```python
from build123d import *

# Parameters (mm, degrees)
F1_DEPTH     = 2.54
F2_T1_DEPTH  = 116.3302767053
F2_T3_DEPTH  = 79.5286740138
F2_T5_DEPTH  = 45.6964583098
F2_T10_DEPTH = 61.1019260212
F2_T15_DEPTH = 53.0222754018
F2_T20_DEPTH = 50.3447363809
F2_T25_DEPTH = 59.0101457163
F2_T31_DEPTH = 50.1034033931
F2_T35_DEPTH = 53.0222754018
F2_T42_DEPTH = 50.3447363809
F2_T46_DEPTH = 48.0116230882


# Not quite as in the source:
# - a fillet or chamfer that OpenCascade refuses, or shapes differently, is made with other operations: its cross-section is extruded or revolved along the edge and cut away or added


with BuildPart() as f1:
    # F0 (on Front) → F1 (new body)
    with BuildSketch(Plane.XZ):
        Polygon((67.8614974022, 19.1138908267), (-26.4717340469, 19.1138908267), (-26.4717340469, -38.417737931), (12.6331467181, -38.417737931), (30.848396942, -38.417737931), (67.8614974022, -38.417737931), align=None)
        Polygon((30.848396942, -38.417737931), (12.6331467181, -38.417737931), (-4.6027889475, -64.2147809267), (19.0966241062, -64.2147809267), align=None)
    extrude(amount=F1_DEPTH)

    # F2: fillet of radius 5.08 on 8 edges, made by hand

    # F2_s2 → F2_t1 (cut)
    with BuildSketch(Plane.YZ.offset(-37.470256675)):
        with BuildLine():
            ThreePointArc((-2.54, 19.1138908267), (-0.6805909488, 17.2544817755), (0, 14.7144817755))
            Line((0, 14.7144817755), (0, 19.1138908267))
            Line((0, 19.1138908267), (-2.54, 19.1138908267))
        make_face()
    extrude(amount=F2_T1_DEPTH, mode=Mode.SUBTRACT)

    # F2_s4 → F2_t3 (cut)
    with BuildSketch(Plane.XY.offset(-49.4162605591)):
        with BuildLine():
            ThreePointArc((-26.4717340469, -2.54), (-24.6123249957, -0.6805909488), (-22.0723249957, 0))
            Line((-22.0723249957, 0), (-26.4717340469, 0))
            Line((-26.4717340469, 0), (-26.4717340469, -2.54))
        make_face()
        with BuildLine():
            ThreePointArc((67.8614974022, -2.54), (66.002088351, -0.6805909488), (63.462088351, 0))
            Line((63.462088351, 0), (67.8614974022, 0))
            Line((67.8614974022, 0), (67.8614974022, -2.54))
        make_face()
    extrude(amount=F2_T3_DEPTH, mode=Mode.SUBTRACT)

    # F2_s6 → F2_t5 (cut)
    with BuildSketch(Plane.YZ.offset(-15.6013115756)):
        with BuildLine():
            ThreePointArc((-2.54, -64.2147809267), (-0.6805909488, -62.3553718755), (0, -59.8153718755))
            Line((0, -59.8153718755), (0, -64.2147809267))
            Line((0, -64.2147809267), (-2.54, -64.2147809267))
        make_face()
    extrude(amount=F2_T5_DEPTH, mode=Mode.SUBTRACT)


with BuildPart() as f2_tool8:
    # F2_s9 → F2_t10 (new body)
    with BuildSketch(Plane.YZ.offset(-37.470256675)):
        with BuildLine():
            ThreePointArc((-2.54, -38.417737931), (-0.6805909488, -36.5583288798), (0, -34.0183288798))
            Line((0, -34.0183288798), (0, -38.417737931))
            Line((0, -38.417737931), (-2.54, -38.417737931))
        make_face()
    extrude(amount=F2_T10_DEPTH)

    split(bisect_by=Plane(origin=(26.480413057, 0, -17.6925198724), x_dir=(0, 1, 0), z_dir=(-0.8314859511, 0, 0.5555457795)), keep=Keep.TOP)


with BuildPart() as f1_1:
    add(f1.part)

    # F2_t7: cut F2_tool8
    add(f2_tool8.part, mode=Mode.SUBTRACT)


with BuildPart() as f2_tool13:
    # F2_s14 → F2_t15 (new body)
    with BuildSketch(Plane(origin=(-7.737083512, 0, -11.5801010106), x_dir=(0, 1, 0), z_dir=(-0.5555457795, 0, -0.8314859511))):
        with BuildLine():
            ThreePointArc((-2.54, 31.8470961801), (-0.6805909488, 33.7065052313), (0, 36.2465052313))
            Line((0, 36.2465052313), (0, 31.8470961801))
            Line((0, 31.8470961801), (-2.54, 31.8470961801))
        make_face()
    extrude(amount=F2_T15_DEPTH)

    split(bisect_by=Plane.XY.offset(-38.417737931), keep=Keep.BOTTOM)


with BuildPart() as f1_2:
    add(f1_1.part)

    # F2_t12: cut F2_tool13
    add(f2_tool13.part, mode=Mode.SUBTRACT)


with BuildPart() as f2_tool18:
    # F2_s19 → F2_t20 (new body)
    with BuildSketch(Plane(origin=(-25.5031201264, 0, -55.983475482), x_dir=(0, 1, 0), z_dir=(0.4145583774, 0, 0.9100227204))):
        with BuildLine():
            ThreePointArc((-2.54, -43.9991372067), (-0.6805909488, -42.1397281555), (0, -39.5997281555))
            Line((0, -39.5997281555), (0, -43.9991372067))
            Line((0, -43.9991372067), (-2.54, -43.9991372067))
        make_face()
    extrude(amount=F2_T20_DEPTH)

    split(bisect_by=Plane.XY.offset(-38.417737931), keep=Keep.BOTTOM)


with BuildPart() as f1_3:
    add(f1_2.part)

    # F2_t17: cut F2_tool18
    add(f2_tool18.part, mode=Mode.SUBTRACT)


with BuildPart() as f2_tool23:
    # F2_s24 → F2_t25 (new body)
    with BuildSketch(Plane.YZ.offset(19.849874314)):
        with BuildLine():
            ThreePointArc((-2.54, -38.417737931), (-0.6805909488, -36.5583288798), (0, -34.0183288798))
            Line((0, -34.0183288798), (0, -38.417737931))
            Line((0, -38.417737931), (-2.54, -38.417737931))
        make_face()
    extrude(amount=F2_T25_DEPTH)

    split(bisect_by=Plane(origin=(40.040214538, 0, -18.2402109276), x_dir=(0, 1, 0), z_dir=(0.9100227204, 0, -0.4145583774)), keep=Keep.TOP)


with BuildPart() as f1_4:
    add(f1_3.part)

    # F2_t22: cut F2_tool23
    add(f2_tool23.part, mode=Mode.SUBTRACT)


with BuildPart() as f2_tool29:
    # F2_s30 → F2_t31 (new body)
    with BuildSketch(Plane.YZ.offset(-26.4717340469)):
        with BuildLine():
            ThreePointArc((-2.54, -38.417737931), (-0.6805909488, -36.5583288798), (0, -34.0183288798))
            Line((0, -34.0183288798), (0, -38.417737931))
            Line((0, -38.417737931), (-2.54, -38.417737931))
        make_face()
    extrude(amount=F2_T31_DEPTH)

    split(bisect_by=Plane(origin=(26.480413057, 0, -17.6925198724), x_dir=(0, 1, 0), z_dir=(0.8314859511, 0, -0.5555457795)), keep=Keep.TOP)


with BuildPart() as f2_tool33:
    # F2_s34 → F2_t35 (new body)
    with BuildSketch(Plane(origin=(-7.737083512, 0, -11.5801010106), x_dir=(0, 1, 0), z_dir=(-0.5555457795, 0, -0.8314859511))):
        with BuildLine():
            ThreePointArc((-2.54, 31.8470961801), (-0.6805909488, 33.7065052313), (0, 36.2465052313))
            Line((0, 36.2465052313), (0, 31.8470961801))
            Line((0, 31.8470961801), (-2.54, 31.8470961801))
        make_face()
    extrude(amount=F2_T35_DEPTH)

    split(bisect_by=Plane.XY.offset(-38.417737931), keep=Keep.TOP)


with BuildPart() as f2_tool29_1:
    add(f2_tool29.part)

    # F2_t37: intersect F2_tool33
    add(f2_tool33.part, mode=Mode.INTERSECT)


with BuildPart() as f1_5:
    add(f1_4.part)

    # F2_t27: cut F2_tool29
    add(f2_tool29_1.part, mode=Mode.SUBTRACT)


with BuildPart() as f2_tool40:
    # F2_s41 → F2_t42 (new body)
    with BuildSketch(Plane(origin=(-25.5031201264, 0, -55.983475482), x_dir=(0, 1, 0), z_dir=(0.4145583774, 0, 0.9100227204))):
        with BuildLine():
            ThreePointArc((-2.54, -43.9991372067), (-0.6805909488, -42.1397281555), (0, -39.5997281555))
            Line((0, -39.5997281555), (0, -43.9991372067))
            Line((0, -43.9991372067), (-2.54, -43.9991372067))
        make_face()
    extrude(amount=F2_T42_DEPTH)

    split(bisect_by=Plane.XY.offset(-38.417737931), keep=Keep.TOP)


with BuildPart() as f2_tool44:
    # F2_s45 → F2_t46 (new body)
    with BuildSketch(Plane.YZ.offset(19.849874314)):
        with BuildLine():
            ThreePointArc((-2.54, -38.417737931), (-0.6805909488, -36.5583288798), (0, -34.0183288798))
            Line((0, -34.0183288798), (0, -38.417737931))
            Line((0, -38.417737931), (-2.54, -38.417737931))
        make_face()
    extrude(amount=F2_T46_DEPTH)

    split(bisect_by=Plane(origin=(40.040214538, 0, -18.2402109276), x_dir=(0, 1, 0), z_dir=(-0.9100227204, 0, 0.4145583774)), keep=Keep.TOP)


with BuildPart() as f2_tool40_1:
    add(f2_tool40.part)

    # F2_t48: intersect F2_tool44
    add(f2_tool44.part, mode=Mode.INTERSECT)


with BuildPart() as f1_6:
    add(f1_5.part)

    # F2_t38: cut F2_tool40
    add(f2_tool40_1.part, mode=Mode.SUBTRACT)


solid = f1_6.part
```
Can you work these out from the model? Positions are in its coordinate system, mm. A direction names the side the tool comes from. Coordinates: 2 decimals unless noted, no trailing zeros. Order: outer loops, then holes, each group sorted by start corner. A loop starts at its lowest first (then second) coordinate and runs counter-clockwise, first axis right, second up. Notation, with made-up numbers: (-7.75, 14) - (11.25, 14) arc R8 ccw to (11.25, 19) - close; hole circle Ø7 at (89, 11.25). An arc over 180 degrees is marked (long way). Answer in a Markdown table with one row per item.
1. Suppose I cut it at B-B (z = -28.5). Please give me the cut outline in (x, y), and give its area (3 significant figures).
Reply:
| item | result |
|---|---|
| outline | (-26.47, -2.54) - (67.86, -2.54) arc R5.08 ccw to (63.46, 0) - (-22.07, 0) arc R5.08 ccw to start |
| area | 233 mm^2 |
2. If I drill on line 1 along Z through (x, y) = (1.5, -2.25); line 2 along Z through (x, y) = (-4, -2.15); line 3 along X through (y, z) = (-0.6, -5.5), over which ranges is the centre line in solid material (lowest first)?
Reply:
| item | result |
|---|---|
| line 1 | z = -64.03 to -55.41, -38.24 to 18.93 |
| line 2 | z = -63.97 to -63.76, -38.17 to 18.86 |
| line 3 | x = -24.47 to 65.86 |
3. If we mould it in two halves opening along Z, with no side actions, what happens to faces 1 (the flat face through (20, 0, -14)), 2 (the cylindrical face through (47.66, -0.7, -36.59)), 3 (the cylindrical face through (7.97, -0.7, -48.68))? For each: pulls with the +Z half, pulls with the -Z half, needs draft (parallel to the pull), parting line crosses it, or undercut.
Reply:
| item | result |
|---|---|
| face 1 | needs draft |
| face 2 | pulls with the -Z half |
| face 3 | undercut |
4. Suppose I cut it at A-A (y = -0.7). Please give me the cut outline in (x, z).
Reply:
| item | result |
|---|---|
| outline | (-24.65, -36.59) - (16.05, -36.59) - (-1.19, -62.39) - (17.92, -62.39) - (29.67, -36.59) - (66.04, -36.59) - (66.04, 17.29) - (-24.65, 17.29) - close |
5. For faces 4 (the cylindrical face through (-3.14, -0.7, -36.59)), 5 (the cylindrical face through (20.03, -0.7, 17.29)), which set-ups out of +Z, -Z, +X, -X, +Y, -Y let a thin tool reach every point of the face, with its end or its side?
Reply:
| item | result |
|---|---|
| face 4 | -X, +Y |
| face 5 | +Z, +X, -X, +Y |
6. For pin 1 (1 mm diameter, centred on y = -1.5, z = -1.5, fed in from -X), with a flat end and sliding along its axis, tell me the tip position at first contact or that it passes through.
Reply:
| item | result |
|---|---|
| pin 1 | stops at x = -26.11 |
7. Suppose I cut it at C-C (x = 52.5). Please give me the cut outline in (y, z).
Reply:
| item | result |
|---|---|
| outline | (-2.54, -38.42) arc R5.08 ccw to (0, -34.02) - (0, 14.71) arc R5.08 ccw to (-2.54, 19.11) - close |
